Input: part model. Units: mm. Frame: model coordinates. Face numbers are marked on the shaded views. A direction names the side the tool comes from. Coordinates: 2 decimals unless noted, no trailing zeros. Write each loop counter-clockwise with the first axis right and the second up, starting at its lowest first coordinate (ties: lowest second). Pieces come first, ordered by that corner, then holes. Notation, with made-up numbers: (-19, -18) - (13, -18) arc R20 cw to (13, -12) - close; hole circle Ø2 at (-26.75, 5.25). An arc over 180 degrees is marked (long way). One line per question, with ' | ' between items. Start each with the question number.
1) Line query: line 1 (Y direction, x = 127, z = -6) (3 decimals); line 2 (Z direction, x = 7, y = 0); line 3 (Y direction, x = 127, z = -3) (3 decimals). Output: solid intervals per line, ascending.
2) Section query A-A on z = -7.5. Return loops of the section in (x, y).
3) Draft query along X for the marked faces 5, 6 and 7. Return one class per face: released by +X, released by -X, zero draft, split by the parting line, or undercut.
4) Reachability of the marked faces 1, 2, 3 and 4 from +Z, -Z, +X, -X, +Y, -Y: full face, straight path, thin tool, end or side. Return the list, or none.
5) Section query B-B on x = 127.5. Return loops of the section in (y, z), and give its area (3 significant figures).
6) Section query D-D on z = 9. Return loops of the section in (x, y), and give its area (3 significant figures).
7) First-contact query: P1, Ø5, axis at x = 111, y = 21.5, coming from the +Z side; P2, Ø15, axis at x = 70.5, z = -13, coming from the +Y side; P3, Ø2, axis at x = 94.5, y = 7, coming from the -Z side. Flat tips, straight axial feed; report the tip coordinate or a pass-through.
8) Section query C-C on y = 57.5. Return loops of the section in (x, z), and give its area (3 significant figures).
```python
from build123d import *

# Parameters (mm, degrees)
BOSS_EXTRUDE1_DEPTH = 17.5
SKETCH3_W           = 47.284329966
SKETCH3_H           = 10
BOSS_EXTRUDE2_DEPTH = 152.5
CUT_EXTRUDE1_DEPTH  = 152.5
SKETCH5_R           = 25
SKETCH5_R_2         = 12.5
BOSS_EXTRUDE3_DEPTH = 15
BOSS_EXTRUDE4_DEPTH = 5
RIB1_REACH          = 178.424
SKETCH7_WALL_W      = 419.848137108
SKETCH7_WALL_H      = 10
FILLET1_R           = 18


with BuildPart() as part:
    # Sketch2 → Boss-Extrude1 (new, symmetric)
    with BuildSketch(Plane(origin=(0, 0, 0), x_dir=(1, 0, 0), z_dir=(0, 1, 0))):
        with BuildLine():
            Line((-20.626994213, -23.642164983), (20.626994213, -23.642164983))
            ThreePointArc((20.626994213, -23.642164983), (37.5, 0), (20.626994213, 23.642164983))
            Line((20.626994213, 23.642164983), (-20.626994213, 23.642164983))
            ThreePointArc((-20.626994213, 23.642164983), (-37.5, 0), (-20.626994213, -23.642164983))
        make_face()
        with BuildLine():
            Line((-18.165876764, -11.142164983), (18.165876764, -11.142164983))
            ThreePointArc((18.165876764, -11.142164983), (25, 0), (18.165876764, 11.142164983))
            Line((18.165876764, 11.142164983), (-18.165876764, 11.142164983))
            ThreePointArc((-18.165876764, 11.142164983), (-25, 0), (-18.165876764, -11.142164983))
        make_face(mode=Mode.SUBTRACT)
    extrude(amount=BOSS_EXTRUDE1_DEPTH, both=True)

    # Sketch3 → Boss-Extrude2 (add)
    with BuildSketch(Plane(origin=(0, 0, 0), x_dir=(0, 0, -1), z_dir=(1, 0, 0))):
        Rectangle(SKETCH3_W, SKETCH3_H)
    extrude(amount=BOSS_EXTRUDE2_DEPTH)

    # Sketch4 → Cut-Extrude1 (cut)
    with BuildSketch(Plane(origin=(0, 17.5, 0), x_dir=(1, 0, 0), z_dir=(0, 1, 0))):
        with BuildLine():
            Line((-18.165876764, -11.142164983), (18.165876764, -11.142164983))
            ThreePointArc((18.165876764, -11.142164983), (25, 0), (18.165876764, 11.142164983))
            Line((18.165876764, 11.142164983), (-18.165876764, 11.142164983))
            ThreePointArc((-18.165876764, 11.142164983), (-25, 0), (-18.165876764, -11.142164983))
        make_face()
    extrude(amount=-CUT_EXTRUDE1_DEPTH, mode=Mode.SUBTRACT)



with BuildPart() as body_2:
    # Sketch5 → Boss-Extrude3 (new, symmetric)
    with BuildSketch(Plane.XY):
        with Locations((127.5, 60.5)):
            Circle(SKETCH5_R)
        with Locations((127.5, 60.5)):
            Circle(SKETCH5_R_2, mode=Mode.SUBTRACT)
    extrude(amount=BOSS_EXTRUDE3_DEPTH, both=True)


with BuildPart() as part_1:
    add(part.part)

    add(body_2.part)  # Boss-Extrude4 merges body 2
    # Sketch6 → Boss-Extrude4 (add, symmetric)
    with BuildSketch(Plane.XY):
        with BuildLine():
            Line((102.5, 60.5), (102.5, 0))
            Line((102.5, 0), (152.5, 0))
            Line((152.5, 0), (152.5, 60.5))
            ThreePointArc((152.5, 60.5), (127.5, 35.5), (102.5, 60.5))
        make_face()
    extrude(amount=BOSS_EXTRUDE4_DEPTH, both=True)

    # Sketch7 wall → Rib1 (add, up to next)
    with BuildSketch(Plane(origin=(70, 13, 0), x_dir=(1, 0, 0), z_dir=(0, 1, 0)), mode=Mode.PRIVATE) as rib1_sk1:
        Rectangle(SKETCH7_WALL_W, SKETCH7_WALL_H)
    rib1_tool1 = extrude(rib1_sk1.sketch, amount=-RIB1_REACH, mode=Mode.PRIVATE) - part_1.part
    add(rib1_tool1.solids().sort_by_distance((70, 13, 0))[0])

    # Fillet1
    fillet1_edges = [part_1.edges().sort_by_distance(p)[0] for p in [
        (102.5, 13, 0),
    ]]
    fillet(fillet1_edges, radius=FILLET1_R)


solid = part_1.part
```
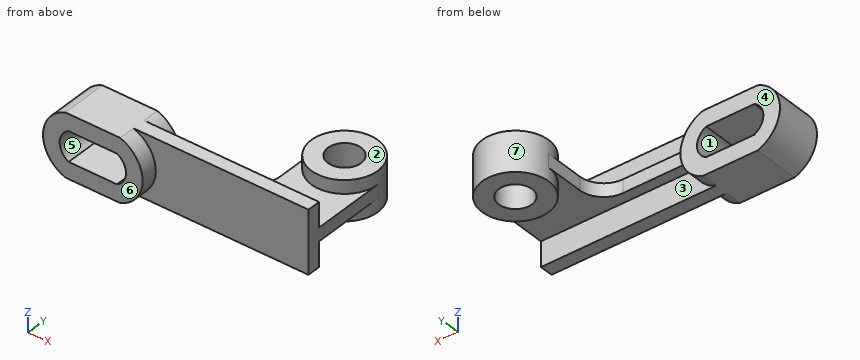
Answer key:
1) line 1: -5 to 5, 35.505 to 48.01, 72.99 to 85.495 | line 2: -23.64 to -11.14, 11.14 to 23.64 | line 3: -5 to 48.01, 72.99 to 85.495
2) outline: (-36.35, -17.5) - (-22.5, -17.5) - (-22.5, 17.5) - (-36.35, 17.5) - close; (22.5, -17.5) - (36.35, -17.5) - (36.35, -5) - (152.5, -5) - (152.5, 5) - (36.35, 5) - (36.35, 17.5) - (22.5, 17.5) - close; circle Ø50 at (127.5, 60.5); hole circle Ø25 at (127.5, 60.5)
3) face 5: undercut | face 6: zero draft | face 7: split by the parting line
4) face 1: +Y, -Y | face 2: +Z, +X, -X, +Y | face 3: -Z, +X | face 4: +Z, -Z, -X, +Y
5) outline: (-5, -23.64) - (5, -23.64) - (5, -5) - (35.5, -5) - (35.5, -15) - (48, -15) - (48, 15) - (35.5, 15) - (35.5, 5) - (5, 5) - (5, 23.64) - (-5, 23.64) - close; (73, -15) - (85.5, -15) - (85.5, 15) - (73, 15) - close | area: 1,530 mm²
6) outline: (-35.82, -17.5) - (-21.17, -17.5) - (-21.17, 17.5) - (-35.82, 17.5) - close; (21.17, -17.5) - (35.82, -17.5) - (35.82, -5) - (152.5, -5) - (152.5, 5) - (35.82, 5) - (35.82, 17.5) - (21.17, 17.5) - close; circle Ø50 at (127.5, 60.5); hole circle Ø25 at (127.5, 60.5) | area: 3,660 mm²
7) P1: z = 5 | P2: y = 5 | P3: z = -5
8) outline: (102.5, -5) - (102.68, -5) - (102.68, -15) - (115.37, -15) - (115.37, 15) - (102.68, 15) - (102.68, 5) - (102.5, 5) - close; (139.63, -15) - (152.32, -15) - (152.32, -5) - (152.5, -5) - (152.5, 5) - (152.32, 5) - (152.32, 15) - (139.63, 15) - close | area: 765 mm²
